```python
from build123d import *

# Parameters (mm, degrees)
ESQUISSE1_W                  = 20
ESQUISSE1_H                  = 20
BOSS_EXTRU_1_DEPTH           = 8
ENL_V_MAT_EXTRU_1_DEPTH      = 9
ESQUISSE4_R                  = 2
ENL_V_MAT_EXTRU_2_DEPTH      = 142.139610307
ENL_V_MAT_EXTRU_2_DEPTH_BACK = 137.139610307
ENL_V_MAT_EXTRU_3_DEPTH      = 9.0000001
ENL_V_MAT_EXTRU_4_DEPTH      = 9
ESQUISSE9_R                  = 2.5
ENL_V_MAT_EXTRU_6_DEPTH      = 9
ENL_V_MAT_EXTRU_8_DEPTH      = 2


with BuildPart() as part:
    # Esquisse1 → Boss.-Extru.1 (new body)
    with BuildSketch(Plane(origin=(0, 0, 0), x_dir=(1, 0, 0), z_dir=(0, 1, 0))):
        with BuildLine():
            Line((-28.284271247, 28.284271247), (70.710678119, 141.421356237))
            ThreePointArc((70.710678119, 141.421356237), (141.421356237, 141.421356237), (141.421356237, 70.710678119))
            Line((141.421356237, 70.710678119), (28.284271247, -28.284271247))
            ThreePointArc((28.284271247, -28.284271247), (-28.284271247, -28.284271247), (-28.284271247, 28.284271247))
        make_face()
        Rectangle(ESQUISSE1_W, ESQUISSE1_H, mode=Mode.SUBTRACT)
    extrude(amount=BOSS_EXTRU_1_DEPTH)

    # Esquisse3 → Enlèv. mat.-Extru.1 (cut, through all)
    with BuildSketch(Plane(origin=(0, 8, 0), x_dir=(1, 0, 0), z_dir=(0, 1, 0))):
        Polygon((-8.232233047, -11.767766953), (-27.234385984, -30.76991989), (-30.76991989, -27.234385984), (-11.767766953, -8.232233047), (-9.726873799, -6.191339893), (-6.191339893, -9.726873799), align=None)
    extrude(amount=-ENL_V_MAT_EXTRU_1_DEPTH, mode=Mode.SUBTRACT)

    # Esquisse4 → Enlèv. mat.-Extru.2 (cut, two sides)
    with BuildSketch(Plane(origin=(1.767766953, 0, 1.767766953), x_dir=(-0.707106781, 0, 0.707106781), z_dir=(-0.707106781, 0, -0.707106781))) as enl_v_mat_extru_2_sk:
        with Locations((34.921798557, 4)):
            Circle(ESQUISSE4_R)
    extrude(amount=ENL_V_MAT_EXTRU_2_DEPTH, mode=Mode.SUBTRACT)
    extrude(enl_v_mat_extru_2_sk.sketch, amount=-ENL_V_MAT_EXTRU_2_DEPTH_BACK, mode=Mode.SUBTRACT)

    # Esquisse5 → Enlèv. mat.-Extru.3 (cut, through all)
    with BuildSketch(Plane(origin=(0, 8, 0), x_dir=(1, 0, 0), z_dir=(0, 1, 0))):
        Polygon((-34.683660608, -14.703220533), (-36.451427561, -16.470987486), (-40.908486709, -7.777625617), (-39.491104164, -6.360243072), (-32.915893655, -12.93545358), align=None)
        Polygon((-7.777625617, -40.908486709), (-6.360243072, -39.491104164), (-12.93545358, -32.915893655), (-14.703220533, -34.683660608), (-16.470987486, -36.451427561), align=None)
    extrude(amount=-ENL_V_MAT_EXTRU_3_DEPTH, mode=Mode.SUBTRACT)

    # Esquisse7 → Enlèv. mat.-Extru.4 (cut, through all)
    with BuildSketch(Plane(origin=(0, 8, 0), x_dir=(1, 0, 0), z_dir=(0, 1, 0))):
        with BuildLine():
            Line((91.923881554, 98.994949366), (102.530483272, 109.601551084))
            ThreePointArc((102.530483272, 109.601551084), (109.601551084, 109.601551084), (109.601551084, 102.530483272))
            Line((109.601551084, 102.530483272), (98.994949366, 91.923881554))
            ThreePointArc((98.994949366, 91.923881554), (91.923881554, 91.923881554), (91.923881554, 98.994949366))
        make_face()
        with BuildLine():
            Line((94.045201898, 119.373629023), (104.651803616, 129.98023074))
            ThreePointArc((104.651803616, 129.98023074), (107.48023074, 129.98023074), (107.48023074, 127.151803616))
            Line((107.48023074, 127.151803616), (96.873629023, 116.545201898))
            ThreePointArc((96.873629023, 116.545201898), (94.045201898, 116.545201898), (94.045201898, 119.373629023))
        make_face()
        with BuildLine():
            Line((71.545201898, 96.873629023), (82.151803616, 107.48023074))
            ThreePointArc((82.151803616, 107.48023074), (84.98023074, 107.48023074), (84.98023074, 104.651803616))
            Line((84.98023074, 104.651803616), (74.373629023, 94.045201898))
            ThreePointArc((74.373629023, 94.045201898), (71.545201898, 94.045201898), (71.545201898, 96.873629023))
        make_face()
        with BuildLine():
            Line((119.373629023, 94.045201898), (129.98023074, 104.651803616))
            ThreePointArc((129.98023074, 104.651803616), (129.98023074, 107.48023074), (127.151803616, 107.48023074))
            Line((127.151803616, 107.48023074), (116.545201898, 96.873629023))
            ThreePointArc((116.545201898, 96.873629023), (116.545201898, 94.045201898), (119.373629023, 94.045201898))
        make_face()
        with BuildLine():
            Line((96.873629023, 71.545201898), (107.48023074, 82.151803616))
            ThreePointArc((107.48023074, 82.151803616), (107.48023074, 84.98023074), (104.651803616, 84.98023074))
            Line((104.651803616, 84.98023074), (94.045201898, 74.373629023))
            ThreePointArc((94.045201898, 74.373629023), (94.045201898, 71.545201898), (96.873629023, 71.545201898))
        make_face()
    extrude(amount=-ENL_V_MAT_EXTRU_4_DEPTH, mode=Mode.SUBTRACT)

    # Esquisse9 → Enlèv. mat.-Extru.6 (cut, through all)
    with BuildSketch(Plane(origin=(0, 0, 0), x_dir=(-1, 0, 0), z_dir=(0, -1, 0))):
        with Locations((-70.710678119, 141.421356237)):
            Circle(ESQUISSE9_R)
        with Locations((-98.244293926, 155.450434208)):
            Circle(ESQUISSE9_R)
        with Locations((-128.765542165, 150.616343387)):
            Circle(ESQUISSE9_R)
        with Locations((-150.616343387, 128.765542165)):
            Circle(ESQUISSE9_R)
        with Locations((-155.450434208, 98.244293926)):
            Circle(ESQUISSE9_R)
        with Locations((-141.421356237, 70.710678119)):
            Circle(ESQUISSE9_R)
        with Locations((-115.287543419, 47.843591903)):
            Circle(ESQUISSE9_R)
    extrude(amount=-ENL_V_MAT_EXTRU_6_DEPTH, mode=Mode.SUBTRACT)

    # Esquisse11 → Enlèv. mat.-Extru.8 (cut)
    with BuildSketch(Plane(origin=(0, 0, 0), x_dir=(-1, 0, 0), z_dir=(0, -1, 0))):
        with BuildLine():
            Line((-88.388347648, 123.743686708), (-77.781745931, 113.13708499))
            ThreePointArc((-77.781745931, 113.13708499), (-77.781745931, 77.781745931), (-113.13708499, 77.781745931))
            Line((-113.13708499, 77.781745931), (-123.743686708, 88.388347648))
            ThreePointArc((-123.743686708, 88.388347648), (-123.743686708, 123.743686708), (-88.388347648, 123.743686708))
        make_face()
    extrude(amount=-ENL_V_MAT_EXTRU_8_DEPTH, mode=Mode.SUBTRACT)


solid = part.part
```
Geometry check sheet. Reference: the model listing, model coordinates, mm. A direction names the side the tool comes from. Round coordinates to 2 decimals unless told otherwise and drop trailing zeros. Order: outer loops, then holes, each group sorted by start corner. A loop starts at its lowest first (then second) coordinate and runs counter-clockwise, first axis right, second up. Notation, with made-up numbers: (4.25, -35) - (26.25, -35) arc R34 ccw to (26.25, -4) - close; hole circle Ø5 at (-23, 2). An arc over 180 degrees is marked (long way). Use a Markdown table: item, result. Add a question column.
1) Section check B-B (x = 50). Record the cut outline in (y, z).
2) Thickness scan on line 1 along Z through (x, y) = (103.5, 7.25); line 2 along Z through (x, y) = (102.5, 5.25); line 3 along Z through (x, y) = (79, 0.5). Record the ranges inside material, lowest first.
3) Section check A-A (z = -1.5). Record the cut outline in (x, y), then the cut area to 3 significant figures.
4) Gauge pin test, flat ends, axial feed: P1, Ø4, axis at x = 3.5, y = 4, coming from the -Z side; P2, Ø1, axis at x = 27.5, y = 6, coming from the -Z side; P3, Ø4, axis at y = 5.5, z = -1, coming from the +X side. Record the tip position at first contact, or that the pin passes through.
5) Set-up check for faces 4 (the flat face through (10, 4, 0)), 5 (the flat face through (107, 2, -94)), 6 (the cylindrical face through (-33.55, 3.94, 21.78)): record each of +Z, -Z, +X, -X, +Y, -Y from which the full face is reachable in a straight line by a thin tool's end or side.
6) Section check C-C (z = -58). Record the cut outline in (x, y).
7) Mould release check, pull along Z, two halves, no side actions. Record for faces 1 (the cylindrical face through (-21.64, 3.94, 33.64)), 2 (the cylindrical face through (141.29, 3.94, -141.55)), 3 (the flat face through (83.159, 0.986, -118.515)): released by +Z, released by -Z, zero draft, split by the parting line, or undercut.
Established:
| question | item | result |
|---|---|---|
| 1 | outline | (0, -117.75) - (8, -117.75) - (8, 9.28) - (0, 9.28) - close |
| 2 | line 1 | -156 to -128.83, -123.17 to -110.36, -96.43 to -83.83, -78.17 to -37.53 |
| 2 | line 2 | -155.94 to -127.83, -122.17 to -109.57, -95.43 to -82.83, -77.17 to -36.65 |
| 2 | line 3 | -148.11 to -114.36, -76.64 to -16.09 |
| 3 | outline | (-39.97, 0) - (-10, 0) - (-10, 8) - (-39.97, 8) - close; (10, 0) - (62.32, 0) - (62.32, 8) - (10, 8) - close |
| 3 | area | 658 mm2 |
| 4 | P1 | z = -66.89 |
| 4 | P2 | z = -92.61 |
| 4 | P3 | x = 64.04 |
| 5 | face 4 | +Y, -Y |
| 5 | face 5 | -Y |
| 5 | face 6 | +Z, -X, +Y, -Y |
| 6 | outline | (-2.28, 0) - (126.89, 0) - (126.89, 8) - (-2.28, 8) - close |
| 7 | face 1 | released by +Z |
| 7 | face 2 | released by -Z |
| 7 | face 3 | undercut |
